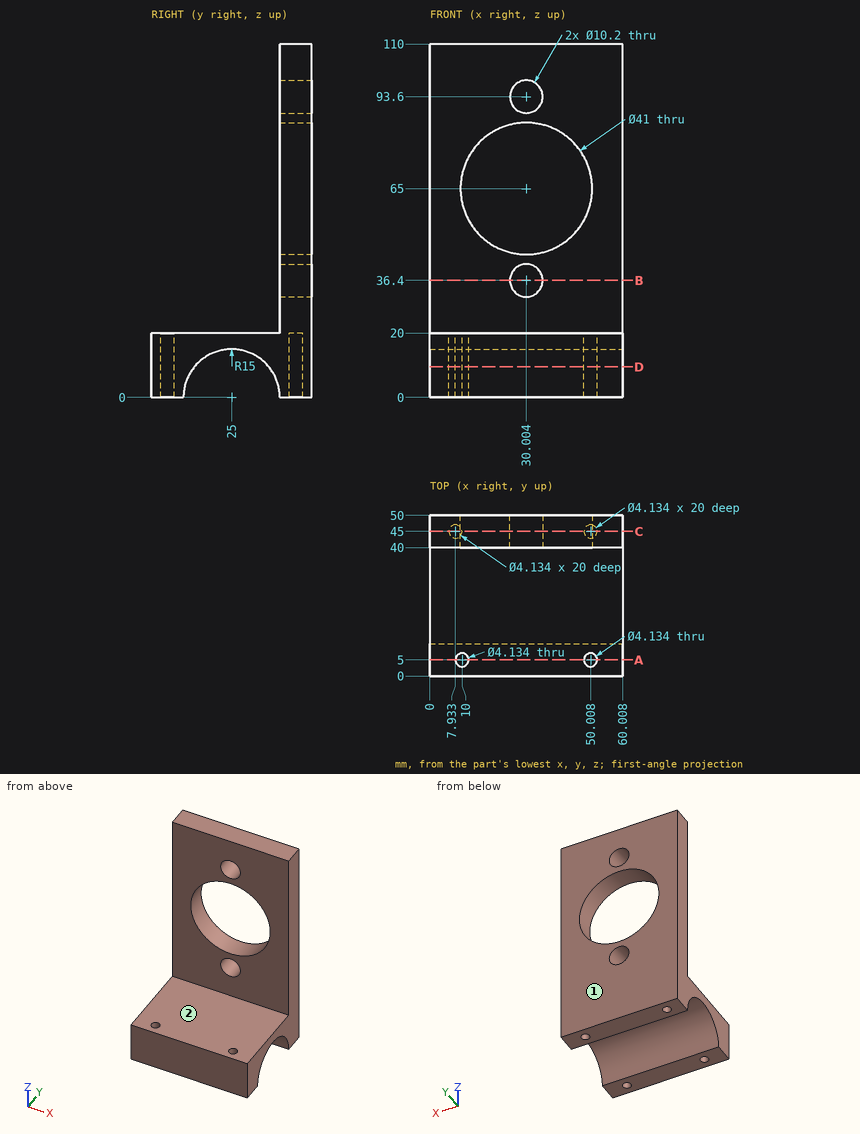
Can you work these out from the drawing? Everything is in mm from the part's minimum corner. A direction names the side the tool comes from. Round coordinates to 2 decimals unless told otherwise and drop trailing zeros. Write each loop counter-clockwise with the first axis right and the second up, starting at its lowest first coordinate (ties: lowest second). Pieces come first, ordered by that corner, then holes. Notation, with made-up numbers: (73.25, -27) - (130.25, -27) arc R32 cw to (130.25, 4) - close; hole circle Ø4 at (3, 24.5). An arc over 180 degrees is marked (long way). Write each question's results on one line, items separated by ' | '. Start each with the question number.
1) Which directions (+Z, -Z, +X, -X, +Y, -Y) give clear straight access to the entire face, cutting with the end or side of a thin tool? Please do the marked faces 1 and 2.
2) Suppose I cut it at D-D (z = 9.5). List the corners of the cut face in (x, y) for me (1 decimal), and give its area (3 significant figures).
3) Suppose I cut it at C-C (y = 45). List the corners of the cut face in (x, z) for me (1 decimal), and give its area (3 significant figures).
4) Please list where these lines run through material, in increasing order: line 1 (X direction, y = 45, z = 6.5) (1 decimal); line 2 (X direction, y = 5, z = 7) (1 decimal); line 3 (X direction, y = 47, z = 36).
5) For pin 1 Ø2 at (x, z) = (6, 59.5) entering from -Y; pin 2 Ø12 at (x, y) = (51, 17) entering from +Z; pin 3 Ø1 at (x, y) = (17, 35.5) entering from -Z, each with a flat end and sliding along its axis, tell me the tip position at first contact or that it passes through.
6) Suppose I cut it at A-A (y = 5). List the corners of the cut face in (x, z) for me (1 decimal).
7) Suppose I cut it at B-B (z = 36.4). List the corners of the cut face in (x, y) for me.
Here are the results:
1) face 1: +Z, -Z, +X, -X, +Y | face 2: +Z, +X, -X, -Y
2) outline: (0, 0) - (60, 0) - (60, 13.4) - (0, 13.4) - close; (0, 36.6) - (60, 36.6) - (60, 50) - (0, 50) - close; hole circle Ø4.1 at (7.9, 45); hole circle Ø4.1 at (10, 5); hole circle Ø4.1 at (50, 5); hole circle Ø4.1 at (50, 45) | area: 1,550 mm2
3) outline: (0, 0) - (5.9, 0) - (5.9, 20) - (10, 20) - (10, 0) - (47.9, 0) - (47.9, 20) - (52.1, 20) - (52.1, 0) - (60, 0) - (60, 110) - (0, 110) - close; hole circle Ø41 at (30, 65); hole circle Ø10.2 at (30, 36.4); hole circle Ø10.2 at (30, 93.6) | area: 4,950 mm2
4) line 1: x = 0 to 5.9, 10 to 47.9, 52.1 to 60 | line 2: x = 0 to 7.9, 12.1 to 47.9, 52.1 to 60 | line 3: x = 0 to 24.92, 35.09 to 60.01
5) pin 1: stops at y = 40 | pin 2: stops at z = 20 | pin 3: stops at z = 10.2
6) outline: (0, 0) - (7.9, 0) - (7.9, 20) - (0, 20) - close; (12.1, 0) - (47.9, 0) - (47.9, 20) - (12.1, 20) - close; (52.1, 0) - (60, 0) - (60, 20) - (52.1, 20) - close
7) outline: (0, 40) - (24.9, 40) - (24.9, 50) - (0, 50) - close; (35.1, 40) - (60.01, 40) - (60.01, 50) - (35.1, 50) - close
